```python
from build123d import *

# Parameters (mm, degrees)
F0_W           = 70
F0_H           = 44
F1_DEPTH       = 27.5
F4_D           = 4.2
F4_DEPTH       = 14.4
F4_TIP         = 1.2618073
F5_D           = 5.5
F5_CBORE_D     = 9.75
F5_CBORE_DEPTH = 12


with BuildPart() as f1:
    # F0 (on Top) → F1 (new body)
    with BuildSketch(Plane.XY):
        Rectangle(F0_W, F0_H)
    extrude(amount=F1_DEPTH)

    # F4
    with Locations(Plane.XY.offset(27.5)):
        with Locations((25, 0), (-25, 0)):
            Hole(F4_D / 2, depth=F4_DEPTH)
            with Locations((0, 0, -(F4_DEPTH + F4_TIP / 2))):  # 118° drill point
                Cone(0, F4_D / 2, F4_TIP, mode=Mode.SUBTRACT)

    # F5 (through all)
    with Locations(Plane.XY.offset(27.5)):
        with Locations((25, -16), (25, 16), (-25, -16), (-25, 16)):
            CounterBoreHole(F5_D / 2, F5_CBORE_D / 2, F5_CBORE_DEPTH)


solid = f1.part
```
For this review, take the finished solid that the model builds, in its own axes (mm). A direction names the side the tool comes from. Coordinates: 2 decimals unless noted, no trailing zeros. Loops run counter-clockwise (first coordinate to the right, second up) from the corner with the lowest first, then second, coordinate; pieces in that order, holes last.
1. Insertion check: P1, Ø5, axis at x = 26, y = 18, coming from the +Z side; P2, Ø3.5, axis at x = -25, y = -16, coming from the +Z side. Each pin has a flat end and moves straight along its axis. Give the tip position at first contact, or say it passes through.
2. For line 1 (Y direction, x = 25, z = 20) (3 decimals); line 2 (X direction, y = 0, z = 19.5); line 3 (X direction, y = -0.5, z = 20.5), list the stretches that pass through material, from the lowest coordinate up.
3. For faces 5 (the flat face through (0, -22, 14)), 6 (the flat face through (27.1, 13.9, 15.5)), list the 3-axis set-ups (+Z, -Z, +X, -X, +Y, -Y) from which the entire face can be reached by the end or side of a thin tool; tool diameter is ignored.
4. Add section A-A, the plane z = 20.5. Give the boundary of the cut face in (x, y) (3 decimals), then the cut area to 3 significant figures.
5. Add section C-C, the plane z = 14.25. Give the boundary of the cut face in (x, y).
6. Add section B-B, the plane y = 16. Give the boundary of the cut face in (x, z) (3 decimals).
7. Mouldability with a two-part tool opening along Y and no side actions: class faces 1 (the flat face through (35, 0, 14)), 2 (the flat face through (0, 22, 14)), 3 (the flat face through (-22.9, 13.9, 15.5)), 4 (the conical face through (24.636, 0.016, 12.057)) as +Y half, -Y half, draft (parallel to the pull), parting line (faces both ways), or undercut.
Result:
1. P1: stops at z = 15.5
1. P2: passes through
2. line 1: y = -22 to -20.875, -11.125 to -2.1, 2.1 to 11.125, 20.875 to 22
2. line 2: x = -35 to -27.1, -22.9 to 22.9, 27.1 to 35
2. line 3: x = -35 to -27.04, -22.96 to 22.96, 27.04 to 35
3. face 5: +Z, -Z, +X, -X, -Y
3. face 6: +Z
4. outline: (-35, -22) - (35, -22) - (35, 22) - (-35, 22) - close; hole circle Ø9.75 at (-25, -16); hole circle Ø9.75 at (-25, 16); hole circle Ø4.2 at (-25, 0); hole circle Ø9.75 at (25, -16); hole circle Ø9.75 at (25, 16); hole circle Ø4.2 at (25, 0)
4. area: 2,750 mm2
5. outline: (-35, -22) - (35, -22) - (35, 22) - (-35, 22) - close; hole circle Ø5.5 at (-25, -16); hole circle Ø5.5 at (-25, 16); hole circle Ø4.2 at (-25, 0); hole circle Ø5.5 at (25, -16); hole circle Ø5.5 at (25, 16); hole circle Ø4.2 at (25, 0)
6. outline: (-35, 0) - (-27.75, 0) - (-27.75, 15.5) - (-29.875, 15.5) - (-29.875, 27.5) - (-35, 27.5) - close; (-22.25, 0) - (22.25, 0) - (22.25, 15.5) - (20.125, 15.5) - (20.125, 27.5) - (-20.125, 27.5) - (-20.125, 15.5) - (-22.25, 15.5) - close; (27.75, 0) - (35, 0) - (35, 27.5) - (29.875, 27.5) - (29.875, 15.5) - (27.75, 15.5) - close
7. face 1: draft
7. face 2: +Y half
7. face 3: undercut
7. face 4: undercut
